CAD build for the part. Positions are in the model's coordinates, mm. A direction names the side the tool comes from. Coordinates: 2 decimals unless noted, no trailing zeros. Order: outer loops, then holes, each group sorted by start corner. A loop starts at its lowest first (then second) coordinate and runs counter-clockwise, first axis right, second up. Notation, with made-up numbers: M 63,73 L 95,73 A21 cw 95,89 Z; hole C 78,13.25 d10. An arc over 180 degrees is marked long. One line per item, written item: value.
from build123d import *

# Parameters (mm, degrees)
SKETCH2_W          = 15.85
SKETCH2_H          = 2.5
FILLET1_R          = 0.762
FILLET2_R          = 0.254
CUT_EXTRUDE1_DEPTH = 6.1


with BuildPart() as part:
    # Sketch1 → Flange (revolve)
    with BuildSketch(Plane(origin=(0, 0, 0), x_dir=(0, 0, -1), z_dir=(1, 0, 0))):
        Polygon((-27.5, 0), (-27.5, 3.175), (-20.315802195, 5.1), (0, 5.1), (0, 2.5), (-20.625, 2.5), (-20.625, 0), align=None)
    revolve(axis=Axis((0, 0, 0), (0, 1, 0)))

    # Sketch2 → Blank Insert (revolve)
    with BuildSketch(Plane(origin=(0, 0, 0), x_dir=(0, 0, -1), z_dir=(1, 0, 0))):
        with Locations((-7.925, 1.25)):
            Rectangle(SKETCH2_W, SKETCH2_H)
    revolve(axis=Axis((0, 0, 0), (0, -1, 0)))

    # Fillet1
    fillet1_edges = [part.edges().sort_by_distance(p)[0] for p in [
        (0, 3.175, -27.5),
    ]]
    fillet(fillet1_edges, radius=FILLET1_R)

    # Fillet2
    fillet2_edges = [part.edges().sort_by_distance(p)[0] for p in [
        (0, 0, -27.5),
    ]]
    fillet(fillet2_edges, radius=FILLET2_R)

    # Sketch3 → Cut-Extrude1 (cut, through all)
    with BuildSketch(Plane(origin=(0, 5.1, 0), x_dir=(1, 0, 0), z_dir=(0, 1, 0))):
        with BuildLine():
            Line((-1.862547623, 6.0198), (1.940673012, 6.0198))
            ThreePointArc((1.940673012, 6.0198), (0.039062695, 13.5128), (-1.862547623, 6.0198))
        make_face()
    cut_extrude1 = extrude(amount=-CUT_EXTRUDE1_DEPTH, mode=Mode.SUBTRACT)

    # Mirror1: Cut-Extrude1 across plane
    add(cut_extrude1.mirror(Plane.XY), mode=Mode.SUBTRACT)


solid = part.part
Q1. Pin check, flat tips, straight feed: pin 1 Ø13 at (x, z) = (0.04, -9.53) entering from +Y; pin 2 Ø1.5 at (x, y) = (5, 1.5) entering from +Z; pin 3 Ø2 at (x, y) = (7.5, 2.5) entering from -Z; pin 4 Ø1.1 at (x, y) = (1, 3) entering from -Z. Stop position of each tip, or through.
Recorded:
pin 1: stops at y = 5.1
pin 2: stops at z = 27.17
pin 3: stops at z = -26.72
pin 4: stops at z = -27.49
Q2. Slice it at A-A (y = 1.75). List the corners of the cut face in (x, z) (3 decimals).
Recorded:
outline: C 0,0 d55; C 0,0 d31.7; hole C 0,0 d41.25; hole M -1.863,-6.02 A3.988 ccw long 1.941,-6.02 Z; hole M -1.863,6.02 L 1.941,6.02 A3.988 ccw long Z
Q3. Drill centre lines: line 1 along X through (y, z) = (2.05, 0) (3 decimals); line 2 along Z through (x, y) = (-2, 0.35); line 3 along X through (y, z) = (1.55, 10.5). Where is each one in solid material? Low to high.
Recorded:
line 1: x = -27.5 to -20.625, -15.85 to 15.85, 20.625 to 27.5
line 2: z = -27.43 to -20.53, -15.72 to -12.95, -6.1 to 6.1, 12.95 to 15.72, 20.53 to 27.43
line 3: x = -25.42 to -17.75, -11.87 to -3.83, 3.91 to 11.87, 17.75 to 25.42
Q4. Slice it at B-B (x = -1). Give the number of separate pieces and of enclosed holes in the cut face, plus the area to 3 significant figures.
Recorded:
separate pieces: 3
enclosed holes: 0
area: 167 mm^2
Q5. Which spindle directions (+Z, -Z, +X, -X, +Y, -Y) get a long thin tool onto all of the face, cutting with end or side? Do faces 1 (the face through (-4.76, 1.27, 15.12)), 2 (the face through (18.3, 0, -10)), 3 (the face through (0, 3, -6.02)). Say none if no direction does.
Recorded:
face 1: -Y
face 2: +Z, -Z, +X, -X, -Y
face 3: +Y, -Y
Q6. Mould opens along X. For faces 4 (the face through (0, 0, 0)), 5 (the face through (0.19, 2.59, -13.51)), 6 (the face through (-26.846, 1.439, -5.961)) say: released by +X, released by -X, zero draft, split by the parting line, or undercut.
Recorded:
face 4: zero draft
face 5: undercut
face 6: split by the parting line
